```python
from build123d import *

# Parameters (mm, degrees)
F1_DEPTH = 76.2
F2_W     = 25.4
F2_H     = 25.4
F3_DEPTH = 12.7
F4_W     = 76.2
F4_H     = 76.2
F6_DEPTH = 25.4
F7_D     = 25.4


with BuildPart() as f1:
    # F0 (on Front) → F1 (new body)
    with BuildSketch(Plane.XZ):
        Polygon((-21.166943, 89.049337), (-21.166943, 17.506457), (-9.800089, 17.506457), (-9.800089, 12.849337), (55.033057, 12.849337), (55.033057, 89.049337), align=None)
    extrude(amount=F1_DEPTH)

    # F2 (on face) → F3 (join)
    with BuildSketch(Plane.XZ.offset(76.2)):
        with Locations((21.700043, 44.061859)):
            Rectangle(F2_W, F2_H)
    extrude(amount=F3_DEPTH)

    # F4 (on face) → F6 (join)
    with BuildSketch(Plane.YZ.offset(55.033057)):
        with Locations((-38.1, 50.949337)):
            Rectangle(F4_W, F4_H)
    extrude(amount=F6_DEPTH)

    # F7 (through all)
    with Locations(Plane.XY.offset(89.049337)):
        with Locations((16.933057, -38.1)):
            Hole(F7_D / 2)


solid = f1.part
```
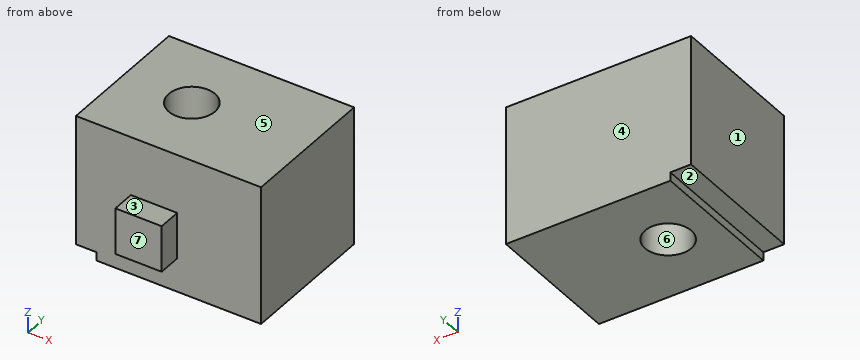
Build history of the part. All positions in model axes, mm. Face numbers are marked on the shaded views. A direction names the side the tool comes from. Give positions to 0.01 mm unless a question says otherwise; leave off trailing zeros. Loops run counter-clockwise (first coordinate to the right, second up) from the corner with the lowest first, then second, coordinate; pieces in that order, holes last. Notation, with made-up numbers: (23.25, 33.5) -> (30.25, 33.5) arc R28 cw to (30.25, 59.5) -> close; hole circle Ø7 at (18, -33.5). An arc over 180 degrees is marked (long way). One line per question, with ' | ' between items. Start each with the question number.
1) Two-plate mould, pull along Y, no slides. Class the marked faces 4, 5, 6 and 7: released by +Y, released by -Y, zero draft, split by the parting line, or undercut.
2) Pin check, flat tips, straight feed: pin 1 (10 mm diameter, centred on y = -85.5, z = 43, fed in from -X); pin 2 (8 mm diameter, centred on x = 38, z = 21, fed in from -Y); pin 3 (10 mm diameter, centred on x = 20, y = -83.5, fed in from -Z); pin 4 (23 mm diameter, centred on x = 16.93, y = -38.1, fed in from -Z). Stop position of each tip, or through.
3) Cut at D-D (x = 66). Give the cut face in (y, z), plus the area to 3 significant figures.
4) Cut at B-B (x = 26). Give the cut face in (y, z).
5) Cut at C-C (z = 61). Give the cut face in (x, y), plus the area to 3 significant figures.
6) 3-axis set-ups, long thin cutter, end or side, ignore diameter. For the marked faces 1, 2 and 3: which of +Z, -Z, +X, -X, +Y, -Y reach the whole face in a straight line?
7) Probe L1, parallel to X at y = -38, z = 30; L2, parallel to Y at x = 40, z = 44; L3, parallel to Y at x = 7, z = 35.5. List the from-to ranges inside material, lowest first.
8) Cut at A-A (y = -38.1). Give the cut face in (x, z).
Return value:
1) face 4: released by +Y | face 5: zero draft | face 6: undercut | face 7: released by -Y
2) pin 1: x = 9 | pin 2: y = -76.2 | pin 3: z = 31.36 | pin 4: through
3) outline: (-76.2, 12.85) -> (0, 12.85) -> (0, 89.05) -> (-76.2, 89.05) -> close | area: 5,810 mm^2
4) outline: (-88.9, 31.36) -> (-76.2, 31.36) -> (-76.2, 12.85) -> (-46.99, 12.85) -> (-46.99, 89.05) -> (-76.2, 89.05) -> (-76.2, 56.76) -> (-88.9, 56.76) -> close; (-29.21, 12.85) -> (0, 12.85) -> (0, 89.05) -> (-29.21, 89.05) -> close
5) outline: (-21.17, -76.2) -> (80.43, -76.2) -> (80.43, 0) -> (-21.17, 0) -> close; hole circle Ø25.4 at (16.93, -38.1) | area: 7,240 mm^2
6) face 1: +Z, -Z, -X, +Y, -Y | face 2: -Z, -X, +Y, -Y | face 3: +Z, +X, -X, -Y
7) L1: -21.17 to 4.23, 29.63 to 80.43 | L2: -76.2 to 0 | L3: -76.2 to -46.01, -30.19 to 0
8) outline: (-21.17, 17.51) -> (-9.8, 17.51) -> (-9.8, 12.85) -> (4.23, 12.85) -> (4.23, 89.05) -> (-21.17, 89.05) -> close; (29.63, 12.85) -> (80.43, 12.85) -> (80.43, 89.05) -> (29.63, 89.05) -> close
